```python
from build123d import *

# Parameters (mm, degrees)
EXTRUDE_1_DEPTH     = 15
SKETCH_2_R          = 2
CUT_EXTRUDE_1_DEPTH = 62
SKETCH_4_R          = 2
CUT_EXTRUDE_2_DEPTH = 62


with BuildPart() as part:
    # 草图1 → 凸台-拉伸1 (new body)
    with BuildSketch(Plane(origin=(0, 0, 0), x_dir=(1, 0, 0), z_dir=(0, 1, 0))):
        with BuildLine():
            Line((-2.142428529, 50.9), (2.142428529, 50.9))
            ThreePointArc((2.142428529, 50.9), (2.672598452, 51.637202321), (2.957914583, 52.49925923))
            Line((2.957914583, 52.49925923), (10.476137794, 52.49925923))
            Line((10.476137794, 52.49925923), (10.094743956, 49.393055687))
            ThreePointArc((10.094743956, 49.393055687), (0, 48.5), (-10.094743956, 49.393055687))
            Line((-10.094743956, 49.393055687), (-10.476137794, 52.49925923))
            Line((-10.476137794, 52.49925923), (-2.957914583, 52.49925923))
            ThreePointArc((-2.957914583, 52.49925923), (-2.672598452, 51.637202321), (-2.142428529, 50.9))
        make_face()
    extrude(amount=EXTRUDE_1_DEPTH)

    # 草图2 → 切除-拉伸1 (cut)
    with BuildSketch(Plane(origin=(-12.821860467, 0, -104.425673493), x_dir=(0.9925461516413212, 0, -0.12186934340515458), z_dir=(0.12186934340515458, 0, 0.9925461516413212))):
        with Locations(Location((0.000150401, 4, 0), (0, 0, 180))):
            Circle(SKETCH_2_R)
        with Locations(Location((0.000150401, 11, 0), (0, 0, 180))):
            Circle(SKETCH_2_R)
    extrude(amount=CUT_EXTRUDE_1_DEPTH, mode=Mode.SUBTRACT)

    # 草图4 → 切除-拉伸2 (cut)
    with BuildSketch(Plane(origin=(12.821860467, 0, -104.425673493), x_dir=(-0.992546151641322, 0, -0.12186934340514766), z_dir=(0.12186934340514766, 0, -0.992546151641322))):
        with Locations((0.000150401, 11)):
            Circle(SKETCH_4_R)
        with Locations((0.000150401, 4)):
            Circle(SKETCH_4_R)
    extrude(amount=-CUT_EXTRUDE_2_DEPTH, mode=Mode.SUBTRACT)


solid = part.part
```
Part model, mm, in its own coordinate system. A direction names the side the tool comes from. Round coordinates to 2 decimals unless told otherwise and drop trailing zeros. Write each loop counter-clockwise with the first axis right and the second up, starting at its lowest first coordinate (ties: lowest second). Pieces come first, ordered by that corner, then holes. Notation, with made-up numbers: (6, 84) -> (35, 84) arc R30 ccw to (35, 121) -> close; hole circle Ø4 at (1.25, 69). An arc over 180 degrees is marked (long way). Return JSON: item names as keys, results as strings. Group by question number.
Q1. Saw through at A-A on y = 10. Write the cut outline in (x, z), plus the area to 3 significant figures.
Q2. Pin check, flat tips, straight feed: pin 1 (2 mm diameter, centred on x = -1.5, y = 5.5, fed in from +Z); pin 2 (3 mm diameter, centred on x = 7.5, y = 13, fed in from +Z); pin 3 (3.5 mm diameter, centred on x = -0.5, y = 4, fed in from -Z). Stop position of each tip, or through.
Q3. Which spindle directions (+Z, -Z, +X, -X, +Y, -Y) get a long thin tool onto all of the face, cutting with end or side? Do faces 1 (the cylindrical face through (0.1, 7.4, -48.5)), 2 (the cylindrical face through (-2.68, 7.4, -51.65)). Say none if no direction does.
Q4. Saw through at C-C on y = 8. Write the cut outline in (x, z), plus the area to 3 significant figures.
Q5. Probe L1, parallel to Y at x = -5.5, z = -49.1; L2, parallel to X at y = 10.5, z = -51.8; L3, parallel to X at y = 11, z = -52.2. List the from-to ranges inside material, lowest first. Write a range as [from, to].
Q6. Mould opens along Y. For faces 3 (the flat face through (10.29, 7.4, -50.97)), 4 (the flat face through (0.1, 15, -50.5)), 5 (the cylindrical face through (4.32, 4.6, -50.84)), 6 (the flat face through (0.1, 0, -50.5)) say: pulls with the +Y half, pulls with the -Y half, needs draft (parallel to the pull), parting line crosses it, or undercut.
Q7. Saw through at B-B on z = -51.35. State how many separate pieces and enclosed holes the cut face has, plus the area to 3 significant figures.
Answer:
{
 "1": {"outline": "(-10.48, -52.5) -> (-8.19, -52.5) -> (-7.76, -49.03) arc R57.5 ccw to (-10.09, -49.39) -> close; (-4.7, -52.5) -> (-2.96, -52.5) arc R3 cw to (-2.14, -50.9) -> (2.14, -50.9) arc R3 cw to (2.96, -52.5) -> (4.7, -52.5) -> (4.23, -48.66) arc R57.5 ccw to (-4.23, -48.66) -> close; (7.76, -49.03) -> (8.19, -52.5) -> (10.48, -52.5) -> (10.09, -49.39) arc R57.5 ccw to start", "area": "41.8 mm2"},
 "2": {"pin 1": "z = -48.5", "pin 2": "z = -48.81", "pin 3": "z = -51.02"},
 "3": {"face 1": "+Z, +Y, -Y", "face 2": "-Z, +Y, -Y"},
 "4": {"outline": "(-10.48, -52.5) -> (-2.96, -52.5) arc R3 cw to (-2.14, -50.9) -> (2.14, -50.9) arc R3 cw to (2.96, -52.5) -> (10.48, -52.5) -> (10.09, -49.39) arc R57.5 ccw to (-10.09, -49.39) -> close", "area": "67.4 mm2"},
 "5": {"L1": "[0, 2.07], [5.93, 9.07], [12.93, 15]", "L2": "[-10.39, -8.31], [-4.41, -2.75], [2.75, 4.41], [8.31, 10.39]", "L3": "[-10.44, -8.42], [-4.39, -2.89], [2.89, 4.39], [8.42, 10.44]"},
 "6": {"face 3": "needs draft", "face 4": "pulls with the +Y half", "face 5": "undercut", "face 6": "pulls with the -Y half"},
 "7": {"separate pieces": "2", "enclosed holes": "4", "area": "184 mm2"}
}
